Could you check a few things on this model? Use its own coordinates, in mm. Coordinates: 2 decimals unless noted, no trailing zeros. Write each loop counter-clockwise with the first axis right and the second up, starting at its lowest first coordinate (ties: lowest second). Pieces come first, ordered by that corner, then holes.
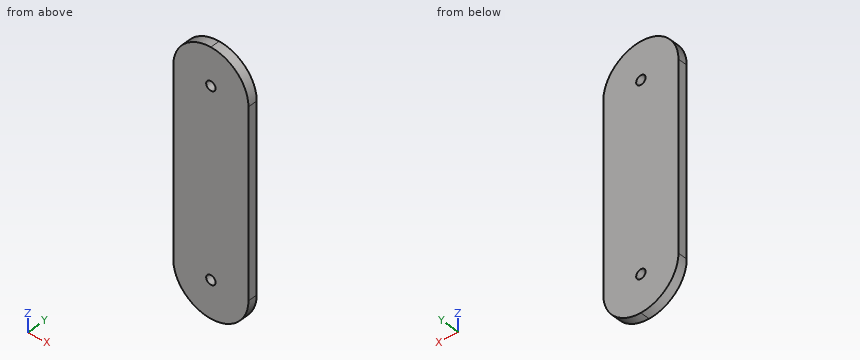
```python
from build123d import *

# Parameters (mm, degrees)
F0_R     = 1.5875
F1_DEPTH = 1.5875


with BuildPart() as f1:
    # F0 (on Front) → F1 (new body, symmetric)
    with BuildSketch(Plane.XZ):
        with BuildLine():
            Line((12.7, -31.75), (12.7, 31.75))
            ThreePointArc((12.7, 31.75), (8.980256, 40.730256), (0, 44.45))
            ThreePointArc((0, 44.45), (-8.980256, 40.730256), (-12.7, 31.75))
            Line((-12.7, 31.75), (-12.7, -31.75))
            ThreePointArc((-12.7, -31.75), (-8.980256, -40.730256), (0, -44.45))
            ThreePointArc((0, -44.45), (8.980256, -40.730256), (12.7, -31.75))
        make_face()
        with Locations((0, -31.75)):
            Circle(F0_R, mode=Mode.SUBTRACT)
        with Locations((0, 31.75)):
            Circle(F0_R, mode=Mode.SUBTRACT)
    extrude(amount=F1_DEPTH, both=True)


solid = f1.part
```
Item 1: I want a section at A-A, the plane y = 0.55. Count the separate pieces of the cut face and the enclosed holes in it, then the cut area to 3 significant figures.
Item 2: Will these pins go through, and if not, where does the flat tip stop? pin 1 Ø1.5 at (x, y) = (-2.5, 0.5) entering from -Z; pin 2 Ø3 at (x, z) = (0, 31.75) entering from -Y.
Item 3: I want a section at B-B, the plane z = -35.5. List the corners of the cut face in (x, y) for me, then the cut area to 3 significant figures.
Item 4: I want a section at C-C, the plane x = 4.25. List the corners of the cut face in (y, z) for me, then the cut area to 3 significant figures.
Item 5: If I drill on line 1 along Z through (x, y) = (-0.75, 0.95); line 2 along Z through (x, y) = (1.25, 0.55); line 3 along Z through (x, y) = (7.5, -0.85), over which ranges is the centre line in solid material (lowest first)?
Taken from the geometry:
1. separate pieces: 1
1. enclosed holes: 2
1. area: 2,100 mm2
2. pin 1: stops at z = -44.33
2. pin 2: passes through
3. outline: (-12.13, -1.59) - (12.13, -1.59) - (12.13, 1.59) - (-12.13, 1.59) - close
3. area: 77.0 mm2
4. outline: (-1.59, -43.72) - (1.59, -43.72) - (1.59, 43.72) - (-1.59, 43.72) - close
4. area: 278 mm2
5. line 1: z = -44.43 to -33.15, -30.35 to 30.35, 33.15 to 44.43
5. line 2: z = -44.39 to -32.73, -30.77 to 30.77, 32.73 to 44.39
5. line 3: z = -42 to 42
